Autodesk Inventor part; units mm, degrees
ref_plane "YZ Plane" through (0, 0, 0) normal (1, 0, 0) x (0, 1, 0)
ref_plane "XZ Plane" through (0, 0, 0) normal (0, 1, 0) x (-1, 0, 0)
ref_plane "XY Plane" through (0, 0, 0) normal (0, 0, 1) x (1, 0, 0)
sketch "Эскиз1" plane through (0, 0, 0) normal (0, 1, 0) x (-1, 0, 0)
  circle A0 centre (15, 10.75) radius 1.75
  circle A1 centre (15, -10.75) radius 1.75
  circle A2 centre (-15, 10.75) radius 1.75
  circle A3 centre (-15, -10.75) radius 1.75
  line L0 (15, 10.75) -> (-15, 10.75) construction
  line L1 (15, 6.75) -> (-15, 6.75)
  line L2 (-15, 14.75) -> (15, 14.75)
  arc A4 (15, 6.75) -> (15, 14.75) centre (15, 10.75) ccw
  arc A5 (-15, 14.75) -> (-15, 6.75) centre (-15, 10.75) ccw
  line L3 (15, -10.75) -> (-15, -10.75) construction
  line L4 (15, -6.75) -> (-15, -6.75)
  line L5 (-15, -14.75) -> (15, -14.75)
  arc A6 (15, -14.75) -> (15, -6.75) centre (15, -10.75) ccw
  arc A7 (-15, -6.75) -> (-15, -14.75) centre (-15, -10.75) ccw
  line L6 (-2.5, -6.75) -> (2.5, -6.75)
  line L7 (2.5, -6.75) -> (2.5, 6.75)
  line L8 (2.5, 6.75) -> (-2.5, 6.75)
  line L9 (-2.5, 6.75) -> (-2.5, -6.75)
  line L10 (-2.5, -6.75) -> (2.5, 6.75) construction
  line L11 (2.5, -6.75) -> (-2.5, 6.75) construction
  point P0 (0, 0)
  point P1 (0, 10.75)
  point P2 (0, -10.75)
  dimension "d0" = 3.5
  dimension "d1" = 21.5
  dimension "d2" = 21.5
  dimension "d3" = 30
  dimension "d4" = 30
  dimension "d5" = 0
  dimension "d6" = 0
  dimension "d7" = 15
  dimension "d8" = 10.75
  dimension "d9" = 30
  dimension "d10" = 4
  dimension "d11" = 30
  dimension "d12" = 4
  dimension "d13" = 5
extrude "Выдавливание1" add sketch "Эскиз1" along normal blind 3
fillet "Сопряжение1" radius 3 4 edges at (-2.5, 1.5, -6.75) (-2.5, 1.5, 6.75) (2.5, 1.5, 6.75) (2.5, 1.5, -6.75)
sketch "Эскиз2" plane through (0, 3, 0) normal (0, 1, 0) x (1, 0, 0)
  line L0 (11, 10.75) -> (7, 10.75) construction
  line L1 (10.5, 11.25) -> (7.5, 11.25)
  line L2 (7.5, 10.25) -> (10.5, 10.25)
  arc A0 (10.5, 10.25) -> (10.5, 11.25) centre (10.5, 10.75) ccw
  arc A1 (7.5, 11.25) -> (7.5, 10.25) centre (7.5, 10.75) ccw
  point P0 (0, 0)
  point P1 (9, 10.75)
  point P2 (15, 10.75)
  dimension "d17" = 1
  dimension "d18" = 3
  dimension "d19" = 0
  dimension "d20" = 4
extrude "Выдавливание2" cut sketch "Эскиз2" against normal blind 3
properties part number "Base"
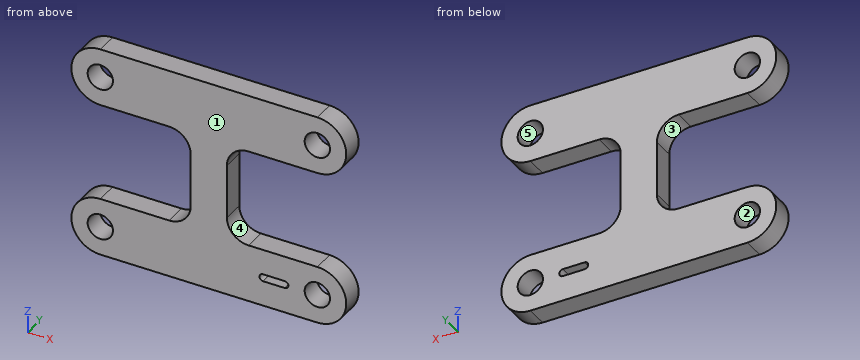
CAD build for the part. Positions are in the model's coordinates, mm. Face numbers are marked on the shaded views. A direction names the side the tool comes from. Coordinates: 2 decimals unless noted, no trailing zeros. Loops run counter-clockwise (first coordinate to the right, second up) from the corner with the lowest first, then second, coordinate; pieces in that order, holes last. Notation, with made-up numbers: (-30, 71) - (-17, 71) arc R13 ccw to (-17, 86) - close; hole circle Ø1 at (68, 23). An arc over 180 degrees is marked (long way). Use one line per item in the form item = value. Start each with the question number.
1) Two-plate mould, pull along Z, no slides. Class the marked faces 1 and 2: +Z half, -Z half, draft (parallel to the pull), parting line (faces both ways), or undercut.
2) Band-saw the part on D-D (x = 14). Give the cut face in (y, z).
3) Flat gauge pin, fed straight in: pin 1 (0.9 mm diameter, centred on y = 2, z = 0, fed in from +X). Where does the tip first touch, or does it go through?
4) Band-saw the part on C-C (z = -10.75). Give the cut face in (x, y).
5) Drill centre lines: L1, parallel to Z at x = -15, y = 2; L2, parallel to Z at x = -11.5, y = 0.75. Where is each one in solid material? Low to high. Write a range as from..to.
6) Band-saw the part on A-A (z = 10.75). Give the cut face in (x, y), and give its area (3 significant figures).
7) Band-saw the part on B-B (x = 8). Give the cut face in (y, z).
8) Tool access for the marked faces 3, 4 and 5: list every direction of +Z, -Z, +X, -X, +Y, -Y with a clear straight run to the whole face (end or side of a thin tool).
Check values:
q1.face_1 = draft
q1.face_2 = undercut
q2.outline = (0, -14.75) - (3, -14.75) - (3, -12.19) - (0, -12.19) - close; (0, -9.31) - (3, -9.31) - (3, -6.75) - (0, -6.75) - close; (0, 6.75) - (3, 6.75) - (3, 9.31) - (0, 9.31) - close; (0, 12.19) - (3, 12.19) - (3, 14.75) - (0, 14.75) - close
q3.pin_1 = 2.5
q4.outline = (-19, 0) - (-16.75, 0) - (-16.75, 3) - (-19, 3) - close; (-13.25, 0) - (7, 0) - (7, 3) - (-13.25, 3) - close; (11, 0) - (13.25, 0) - (13.25, 3) - (11, 3) - close; (16.75, 0) - (19, 0) - (19, 3) - (16.75, 3) - close
q5.L1 = -14.75..-12.5, -9..-6.75, 6.75..9, 12.5..14.75
q5.L2 = -14.75..-6.75, 6.75..14.75
q6.outline = (-19, 0) - (-16.75, 0) - (-16.75, 3) - (-19, 3) - close; (-13.25, 0) - (13.25, 0) - (13.25, 3) - (-13.25, 3) - close; (16.75, 0) - (19, 0) - (19, 3) - (16.75, 3) - close
q6.area = 93.0 mm2
q7.outline = (0, -14.75) - (3, -14.75) - (3, -11.25) - (0, -11.25) - close; (0, -10.25) - (3, -10.25) - (3, -6.75) - (0, -6.75) - close; (0, 6.75) - (3, 6.75) - (3, 14.75) - (0, 14.75) - close
q8.face_3 = -X, +Y, -Y
q8.face_4 = +X, +Y, -Y
q8.face_5 = +Y, -Y
